Check sheet for the modelled part. Datum: model origin and axes. Units: mm. A direction names the side the tool comes from. Round coordinates to 2 decimals unless told otherwise and drop trailing zeros. Write each loop counter-clockwise with the first axis right and the second up, starting at its lowest first coordinate (ties: lowest second). Pieces come first, ordered by that corner, then holes.
Item 1: Section check B-B, the plane z = -0.75. Record the cut outline in (x, y).
Item 2: Section check A-A, the plane x = 0. Record the cut outline in (y, z).
Item 3: Depth check by flat-ended pin: pin 1 (2 mm diameter, centred on x = 6, z = -0.5, fed in from -Y); pin 2 (2 mm diameter, centred on x = -13.5, z = 1, fed in from -Y); pin 3 (1.5 mm diameter, centred on y = -3.5, z = -2, fed in from +X). Enter the tip coordinate at first touch or a pass-through.
Item 4: Material ranges on line 1 along Z through (x, y) = (4.5, 2); line 2 along X through (y, z) = (5.5, 0.5); line 3 along Y through (x, z) = (0, 4.25), recorded low to high.
Item 5: Section check D-D, the plane y = -7. Record the cut outline in (x, z) (1 decimal).
Item 6: Section check C-C, the plane y = 13. Record the cut outline in (x, z), plus the area to 3 significant figures.
Item 7: Release check for a two-part mould opening along X. For faces 1 (the flat face through (-20, 7, 0)), 2 (the flat face through (0, 0, 1.5)), 3 (the flat face through (0, 15, 2)) record: pulls with the +X half, pulls with the -X half, needs draft (parallel to the pull), parting line crosses it, or undercut.
Item 8: Set-up check for faces 4 (the flat face through (-16, 7, 0)), 5 (the cylindrical face through (0, -20, 0)): record each of +Z, -Z, +X, -X, +Y, -Y from which the full face is reachable in a straight line by a thin tool's end or side.
from build123d import *

# Parameters (mm, degrees)
EXTRUDE_1_DEPTH     = 5
CUT_EXTRUDE_2_DEPTH = 1.5


with BuildPart() as part:
    # 草图1 → 凸台-拉伸1 (new, symmetric)
    with BuildSketch(Plane.XY):
        with BuildLine():
            Line((-20, 0), (-20, 15))
            Line((-20, 15), (20, 15))
            Line((20, 15), (20, 0))
            ThreePointArc((20, 0), (0, -20), (-20, 0))
        make_face()
    extrude(amount=EXTRUDE_1_DEPTH, both=True)

    # 草图2 → 切除-拉伸2 (cut, symmetric)
    with BuildSketch(Plane.XY):
        with BuildLine():
            Line((-16, 0), (-16, 15))
            Line((-16, 15), (16, 15))
            Line((16, 15), (16, 0))
            ThreePointArc((16, 0), (0, -16), (-16, 0))
        make_face()
    extrude(amount=CUT_EXTRUDE_2_DEPTH, both=True, mode=Mode.SUBTRACT)


solid = part.part
Values found:
1. outline: (-20, 0) arc R20 ccw to (20, 0) - (20, 15) - (16, 15) - (16, 0) arc R16 cw to (-16, 0) - (-16, 15) - (-20, 15) - close
2. outline: (-20, -5) - (15, -5) - (15, -1.5) - (-16, -1.5) - (-16, 1.5) - (15, 1.5) - (15, 5) - (-20, 5) - close
3. pin 1: stops at y = -19.36
3. pin 2: stops at y = -15.61
3. pin 3: stops at x = 19.81
4. line 1: z = -5 to -1.5, 1.5 to 5
4. line 2: x = -20 to -16, 16 to 20
4. line 3: y = -20 to 15
5. outline: (-18.7, -5) - (18.7, -5) - (18.7, 5) - (-18.7, 5) - close; hole (-14.4, -1.5) - (14.4, -1.5) - (14.4, 1.5) - (-14.4, 1.5) - close
6. outline: (-20, -5) - (20, -5) - (20, 5) - (-20, 5) - close; hole (-16, -1.5) - (16, -1.5) - (16, 1.5) - (-16, 1.5) - close
6. area: 304 mm2
7. face 1: pulls with the -X half
7. face 2: undercut
7. face 3: needs draft
8. face 4: +Y
8. face 5: +Z, -Z, -Y
